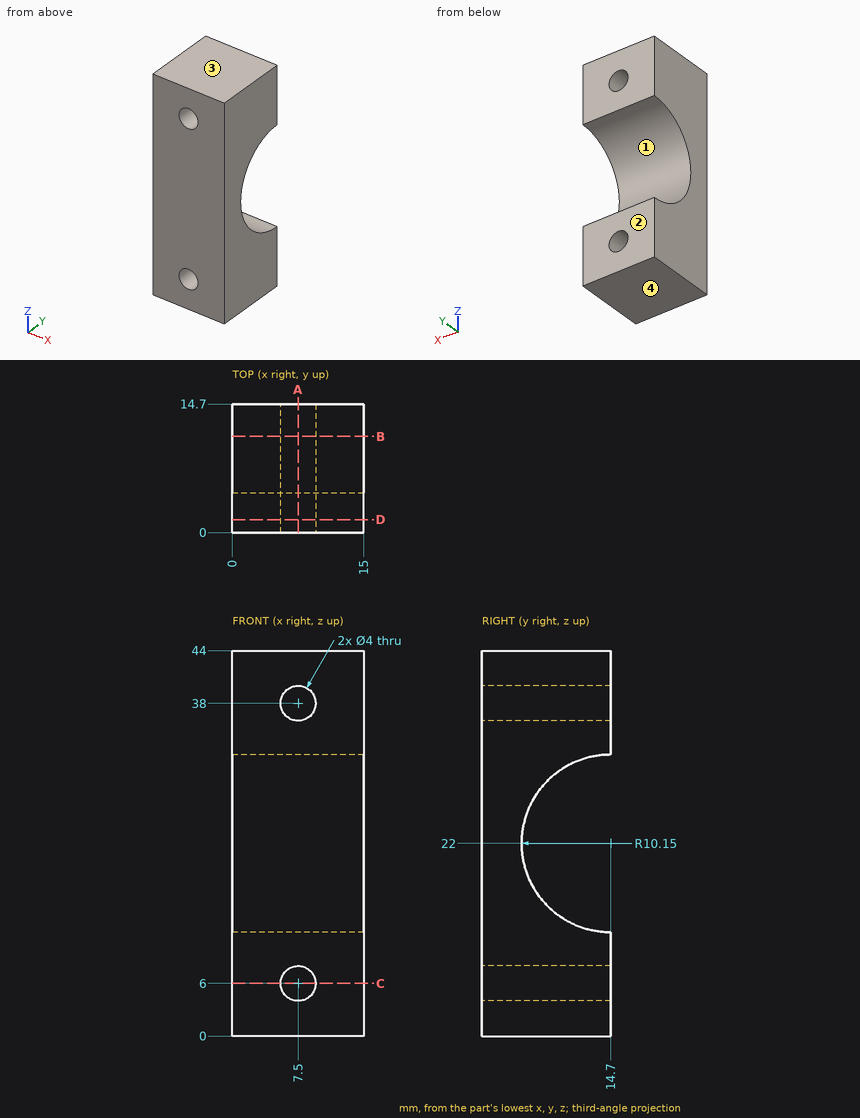
For this review, use the dimensioned drawing (mm, ordinates from the lowest corner) and the shaded views. Give positions to 0.01 mm unless a question says otherwise; leave off trailing zeros. Order: outer loops, then holes, each group sorted by start corner. A loop starts at its lowest first (then second) coordinate and runs counter-clockwise, first axis right, second up.
1) The part is to be moulded in two halves that separate along Z. For the marked faces 1, 2, 3 and 4, say which applies: released by +Z, released by -Z, zero draft, split by the parting line, or undercut.
2) Take a section at C-C (z = 6). Give the boundary of the cut face in (x, y), then the cut area to 3 significant figures.
3) Take a section at D-D (y = 1.5). Give the boundary of the cut face in (x, z).
4) Wall thickness on line 1 (Z direction, x = 7.5, y = 6); line 2 (Z direction, x = 6.5, y = 4.5); line 3 (Z direction, x = 4, y = 7): over which ranges is each line inside the solid? List them lowest first.
5) Take a section at A-A (x = 7.5). Give the boundary of the cut face in (y, z).
6) Take a section at B-B (y = 11). Give the boundary of the cut face in (x, z), then the cut area to 3 significant figures.
7) Insertion check: pin 1 (1 mm diameter, centred on y = 9.5, z = 16, fed in from -X). The pin has a flat end and moves straight along its axis. Give the tip position at first contact, or say it passes through.
Derived:
1. face 1: undercut
1. face 2: zero draft
1. face 3: released by +Z
1. face 4: released by -Z
2. outline: (0, 0) - (5.5, 0) - (5.5, 14.7) - (0, 14.7) - close; (9.5, 0) - (15, 0) - (15, 14.7) - (9.5, 14.7) - close
2. area: 162 mm2
3. outline: (0, 0) - (15, 0) - (15, 44) - (0, 44) - close; hole circle Ø4 at (7.5, 6); hole circle Ø4 at (7.5, 38)
4. line 1: z = 0 to 4, 8 to 16.77, 27.23 to 36, 40 to 44
4. line 2: z = 0 to 4.27, 7.73 to 36.27, 39.73 to 44
4. line 3: z = 0 to 15.39, 28.61 to 44
5. outline: (0, 0) - (14.7, 0) - (14.7, 4) - (0, 4) - close; (0, 8) - (14.7, 8) - (14.7, 11.85) arc R10.15 cw to (14.7, 32.15) - (14.7, 36) - (0, 36) - close; (0, 40) - (14.7, 40) - (14.7, 44) - (0, 44) - close
6. outline: (0, 0) - (15, 0) - (15, 12.55) - (0, 12.55) - close; (0, 31.45) - (15, 31.45) - (15, 44) - (0, 44) - close; hole circle Ø4 at (7.5, 6); hole circle Ø4 at (7.5, 38)
6. area: 351 mm2
7. pin 1: passes through
